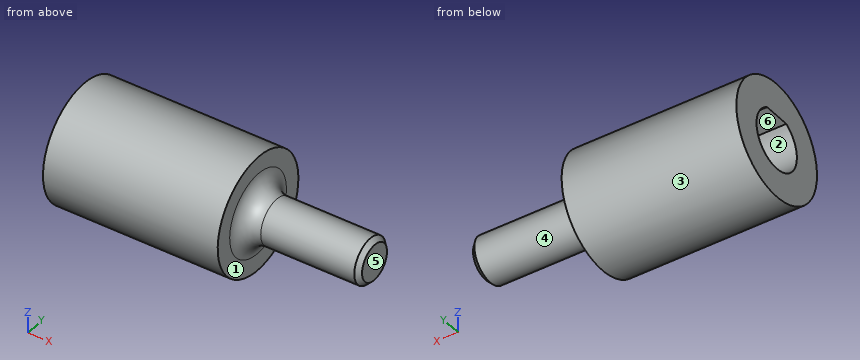
from build123d import *

# Parameters (mm, degrees)
CONG_1_R                = 2
ENL_V_MAT_EXTRU_1_DEPTH = 15.875
CHANFREIN1_SIZE         = 0.5


with BuildPart() as part:
    # Esquisse3 → Révolution1 (revolve)
    with BuildSketch(Plane(origin=(0, 0, 0), x_dir=(1, 0, 0), z_dir=(0, 1, 0)), mode=Mode.PRIVATE) as r_volution1_sk:
        Polygon((0, 6.35), (19.05, 6.35), (19.05, 2.4638), (31.75, 2.4638), (31.75, 0), (0, 0), align=None)
    revolve(r_volution1_sk.sketch.rotate(Axis((0, 0, 0), (1, 0, 0)), 180), axis=Axis((0, 0, 0), (1, 0, 0)))

    # Congé1
    cong_1_edges = [part.edges().sort_by_distance(p)[0] for p in [
        (19.05, 0, -2.4638),
    ]]
    fillet(cong_1_edges, radius=CONG_1_R)

    # Esquisse4 → Enlèv. mat.-Extru.1 (cut)
    with BuildSketch(Plane.ZY):
        with BuildLine():
            Line((2.794, -1.508041445), (2.794, 1.508041445))
            ThreePointArc((2.794, 1.508041445), (-3.175, 0), (2.794, -1.508041445))
        make_face()
    extrude(amount=-ENL_V_MAT_EXTRU_1_DEPTH, mode=Mode.SUBTRACT)

    # Chanfrein1
    chanfrein1_edges = [part.edges().sort_by_distance(p)[0] for p in [
        (31.75, 0, -2.4638),
    ]]
    chamfer(chanfrein1_edges, length=CHANFREIN1_SIZE)


solid = part.part
For this review, take the finished solid that the model builds, in its own axes (mm). Face numbers are marked on the shaded views. A direction names the side the tool comes from. Round coordinates to 2 decimals unless told otherwise and drop trailing zeros. Order: outer loops, then holes, each group sorted by start corner. A loop starts at its lowest first (then second) coordinate and runs counter-clockwise, first axis right, second up. Notation, with made-up numbers: (45.5, 79.5) -> (56.5, 79.5) arc R22 ccw to (56.5, 85.5) -> close; hole circle Ø8 at (75.25, 29). An arc over 180 degrees is marked (long way). Put each result on its own line as item: value.
Q1. Add section C-C on y = 0. Write out the cut boundary in (x, z) (3 decimals).
Check result:
outline: (0, -6.35) -> (19.05, -6.35) -> (19.05, -4.464) arc R2 cw to (21.05, -2.464) -> (31.25, -2.464) -> (31.75, -1.964) -> (31.75, 1.964) -> (31.25, 2.464) -> (21.05, 2.464) arc R2 cw to (19.05, 4.464) -> (19.05, 6.35) -> (0, 6.35) -> (0, 2.794) -> (15.875, 2.794) -> (15.875, -3.175) -> (0, -3.175) -> close
Q2. Add section D-D on x = 23. Write out the cut boundary in (y, z).
Check result:
outline: circle Ø4.93 at (0, 0)
Q3. Machinability: for the marked faces 4, 5 and 6, which of the approach directions +Z, -Z, +X, -X, +Y, -Y give a long, thin tool a straight path to every point of the face, cutting with its end or side? Answer none if there is none.
Check result:
face 4: +X
face 5: +Z, -Z, +X, +Y, -Y
face 6: -X
Q4. For probe 1 along Y at (x, z) = (12, 0) (3 decimals); probe 2 along X at (y, z) = (-3, -3.75); probe 3 along Y at (x, z) = (9.5, -1.5), list the stretches that pass through material, from the lowest coordinate up. Write a range as [from, to].
Check result:
probe 1: [-6.35, -3.175], [3.175, 6.35]
probe 2: [0, 19.05]
probe 3: [-6.17, -2.8], [2.8, 6.17]
Q5. Insertion check: pin 1 Ø1 at (y, z) = (1, -3.5) entering from -X; pin 2 Ø4 at (x, z) = (22.5, -1) entering from -Y; pin 3 Ø1 at (x, y) = (4, -4) entering from -Z; pin 4 Ø4 at (x, y) = (26, 5) entering from -Z. Each pin has a flat end and moves straight along its axis. Give the tip position at first contact, or say it passes through.
Check result:
pin 1: x = 0
pin 2: y = -2.49
pin 3: z = -5.3
pin 4: through
Q6. Mouldability with a two-part tool opening along Z and no side actions: class the marked faces 1, 2 and 3 as pulls with the +Z half, pulls with the -Z half, needs draft (parallel to the pull), parting line crosses it, or undercut.
Check result:
face 1: needs draft
face 2: undercut
face 3: parting line crosses it
Q7. Add section A-A on z = 0. Write out the cut boundary in (x, y) (3 decimals), plus the area to 3 significant figures.
Check result:
outline: (0, -6.35) -> (19.05, -6.35) -> (19.05, -4.464) arc R2 cw to (21.05, -2.464) -> (31.25, -2.464) -> (31.75, -1.964) -> (31.75, 1.964) -> (31.25, 2.464) -> (21.05, 2.464) arc R2 cw to (19.05, 4.464) -> (19.05, 6.35) -> (0, 6.35) -> (0, 3.175) -> (15.875, 3.175) -> (15.875, -3.175) -> (0, -3.175) -> close
area: 205 mm2
Q8. Add section B-B on x = 15.5. Write out the cut boundary in (y, z) (3 decimals).
Check result:
outline: circle Ø12.7 at (0, 0); hole (-1.508, 2.794) arc R3.175 ccw (long way) to (1.508, 2.794) -> close
